Geometry: see drawing. Coordinates: mm, zero at the bounding-box minimum. A direction names the side the tool comes from. Round coordinates to 2 decimals unless told otherwise and drop trailing zeros. Write each loop counter-clockwise with the first axis right and the second up, starting at its lowest first coordinate (ties: lowest second). Pieces come first, ordered by that corner, then holes.
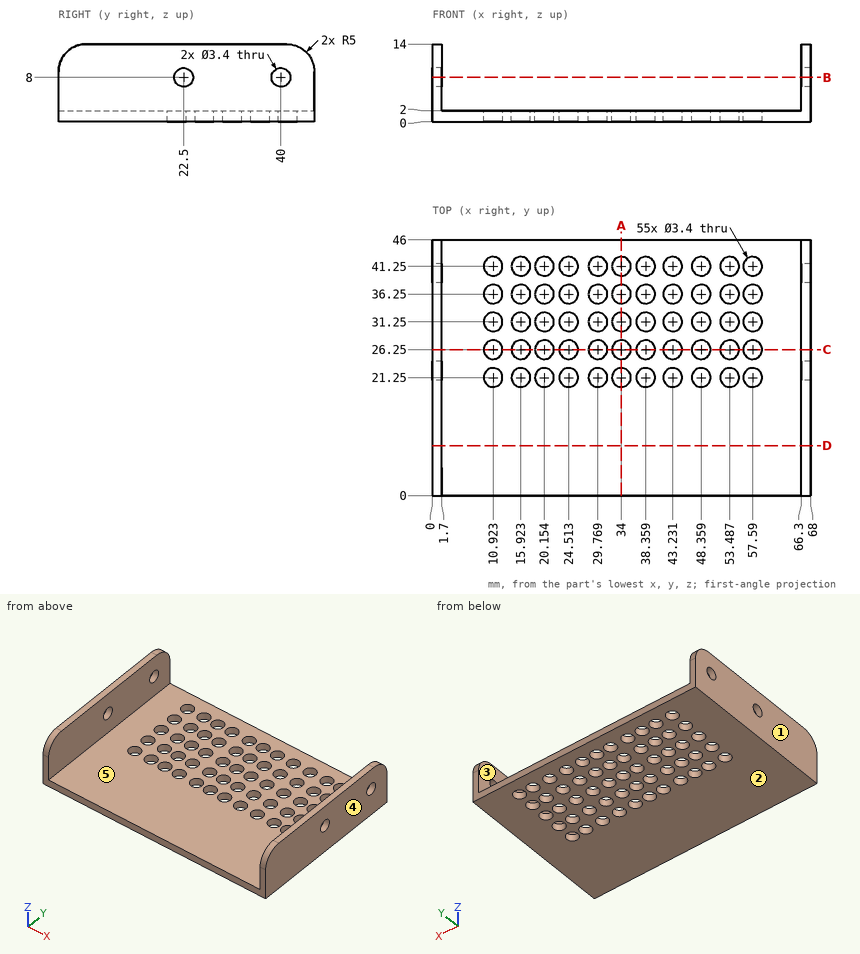
1) Material intervals for line 1 (X direction, y = 24, z = 10.75); line 2 (Z direction, x = 23.5, y = 29), sorted ascending.
Taken from the geometry:
line 1: x = 0 to 1.7, 66.3 to 68
line 2: z = 0 to 2
2) Section query A-A on x = 34. Return the cut outline in (y, z), then the cut area to 3 significant figures.
Taken from the geometry:
outline: (0, 0) - (19.55, 0) - (19.55, 2) - (0, 2) - close; (22.95, 0) - (24.55, 0) - (24.55, 2) - (22.95, 2) - close; (27.95, 0) - (29.55, 0) - (29.55, 2) - (27.95, 2) - close; (32.95, 0) - (34.55, 0) - (34.55, 2) - (32.95, 2) - close; (37.95, 0) - (39.55, 0) - (39.55, 2) - (37.95, 2) - close; (42.95, 0) - (46, 0) - (46, 2) - (42.95, 2) - close
area: 58.0 mm2
3) Contact query for flat-ended pins moving along their axis: P1, Ø3, axis at x = 57.59, y = 21.25, coming from the +Z side; P2, Ø4.5, axis at x = 57.59, y = 26.25, coming from the +Z side. Output: stop coordinate, or through.
Taken from the geometry:
P1: passes through
P2: stops at z = 2
4) Pull-direction query (X, two-part tool) for the marked faces 1, 2 and 3; classes: released by +X, released by -X, zero draft, split by the parting line, or undercut.
Taken from the geometry:
face 1: released by -X
face 2: zero draft
face 3: undercut
5) Section query C-C on y = 26.25. State how many separate pieces and enclosed holes the cut face has, then the cut area to 3 significant figures.
Taken from the geometry:
separate pieces: 12
enclosed holes: 0
area: 102 mm2
6) Section query D-D on y = 9. Return the cut outline in (x, z), then the cut area to 3 significant figures.
Taken from the geometry:
outline: (0, 0) - (68, 0) - (68, 14) - (66.3, 14) - (66.3, 2) - (1.7, 2) - (1.7, 14) - (0, 14) - close
area: 177 mm2
7) Reachability of the marked faces 4 and 5 from +Z, -Z, +X, -X, +Y, -Y: full face, straight path, thin tool, end or side. Return the list, or none.
Taken from the geometry:
face 4: +Z, -Z, +X, +Y, -Y
face 5: +Z, +Y, -Y
8) Section query B-B on z = 8. Return the cut outline in (x, y).
Taken from the geometry:
outline: (0, 0) - (1.7, 0) - (1.7, 20.8) - (0, 20.8) - close; (0, 24.2) - (1.7, 24.2) - (1.7, 38.3) - (0, 38.3) - close; (0, 41.7) - (1.7, 41.7) - (1.7, 46) - (0, 46) - close; (66.3, 0) - (68, 0) - (68, 20.8) - (66.3, 20.8) - close; (66.3, 24.2) - (68, 24.2) - (68, 38.3) - (66.3, 38.3) - close; (66.3, 41.7) - (68, 41.7) - (68, 46) - (66.3, 46) - close
